```python
from build123d import *

# Parameters (mm, degrees)
F0_W      = 800
F0_H      = 300
F0_H_2    = 200
F1_DEPTH  = 100
F2_R      = 25
F2_R_2    = 75
F3_DEPTH  = 100
F4_R      = 75
F5_DEPTH  = 150
F6_R      = 82.5
F6_R_2    = 9
F6_R_3    = 25
F7_DEPTH  = 25
F8_R      = 50
F8_R_2    = 25
F9_DEPTH  = 5
F10_R     = 75
F11_DEPTH = 25
F12_R     = 37.5
F13_DEPTH = 100
F14_R     = 92.5
F14_R_2   = 9
F14_R_3   = 37.5
F15_DEPTH = 25
F16_R     = 60
F16_R_2   = 37.5
F17_DEPTH = 5
F18_W     = 1200
F18_H     = 1000
F19_DEPTH = 100
F20_W     = 1400
F20_H     = 100
F21_DEPTH = 100
F23_DEPTH = 100


with BuildPart() as f1:
    # F0 (on Front) → F1 (new body)
    with BuildSketch(Plane.XZ):
        Polygon((400, -965), (550, -965), (550, 965), (-550, 965), (-550, -965), (-400, -965), (-400, -765), (400, -765), align=None)
        with Locations((0, -465)):
            Rectangle(F0_W, F0_H, mode=Mode.SUBTRACT)
        with Locations((0, -65)):
            Rectangle(F0_W, F0_H_2, mode=Mode.SUBTRACT)
    extrude(amount=F1_DEPTH)

    # F2 (on face) → F3 (cut)
    with BuildSketch(Plane.XZ.offset(100)):
        with Locations((-300, 125)):
            Circle(F2_R)
        with Locations((0, 425)):
            Circle(F2_R_2)
        with Locations((-300, 725)):
            Circle(F2_R)
        with Locations((300, 125)):
            Circle(F2_R)
        with Locations((300, 725)):
            Circle(F2_R)
    extrude(amount=-F3_DEPTH, mode=Mode.SUBTRACT)

    # F4 (on face) → F5 (join)
    with BuildSketch(Plane.XZ.offset(100)):
        with Locations((-455, 425)):
            Circle(F4_R)
        with Locations((455, 425)):
            Circle(F4_R)
    extrude(amount=F5_DEPTH)

    # F6 (on face) → F7 (join)
    with BuildSketch(Plane.XZ.offset(100)):
        with Locations((-300, 725)):
            Circle(F6_R)
        with Locations((-300, 662.5)):
            Circle(F6_R_2, mode=Mode.SUBTRACT)
        with Locations((-362.5, 725)):
            Circle(F6_R_2, mode=Mode.SUBTRACT)
        with Locations((-300, 725)):
            Circle(F6_R_3, mode=Mode.SUBTRACT)
        with Locations((-300, 787.5)):
            Circle(F6_R_2, mode=Mode.SUBTRACT)
        with Locations((-237.5, 725)):
            Circle(F6_R_2, mode=Mode.SUBTRACT)
        with Locations((-300, 125)):
            Circle(F6_R)
        with Locations((-300, 62.5)):
            Circle(F6_R_2, mode=Mode.SUBTRACT)
        with Locations((-362.5, 125)):
            Circle(F6_R_2, mode=Mode.SUBTRACT)
        with Locations((-300, 125)):
            Circle(F6_R_3, mode=Mode.SUBTRACT)
        with Locations((-237.5, 125)):
            Circle(F6_R_2, mode=Mode.SUBTRACT)
        with Locations((-300, 187.5)):
            Circle(F6_R_2, mode=Mode.SUBTRACT)
        with Locations((300, 725)):
            Circle(F6_R)
        with Locations((300, 662.5)):
            Circle(F6_R_2, mode=Mode.SUBTRACT)
        with Locations((237.5, 725)):
            Circle(F6_R_2, mode=Mode.SUBTRACT)
        with Locations((300, 725)):
            Circle(F6_R_3, mode=Mode.SUBTRACT)
        with Locations((362.5, 725)):
            Circle(F6_R_2, mode=Mode.SUBTRACT)
        with Locations((300, 787.5)):
            Circle(F6_R_2, mode=Mode.SUBTRACT)
        with Locations((300, 125)):
            Circle(F6_R)
        with Locations((237.5, 125)):
            Circle(F6_R_2, mode=Mode.SUBTRACT)
        with Locations((300, 62.5)):
            Circle(F6_R_2, mode=Mode.SUBTRACT)
        with Locations((300, 125)):
            Circle(F6_R_3, mode=Mode.SUBTRACT)
        with Locations((362.5, 125)):
            Circle(F6_R_2, mode=Mode.SUBTRACT)
        with Locations((300, 187.5)):
            Circle(F6_R_2, mode=Mode.SUBTRACT)
    extrude(amount=F7_DEPTH)

    # F8 (on face) → F9 (join)
    with BuildSketch(Plane.XZ.offset(125)):
        with Locations((-300, 725)):
            Circle(F8_R)
        with Locations((-300, 725)):
            Circle(F8_R_2, mode=Mode.SUBTRACT)
        with Locations((-300, 125)):
            Circle(F8_R)
        with Locations((-300, 125)):
            Circle(F8_R_2, mode=Mode.SUBTRACT)
        with Locations((300, 725)):
            Circle(F8_R)
        with Locations((300, 725)):
            Circle(F8_R_2, mode=Mode.SUBTRACT)
        with Locations((300, 125)):
            Circle(F8_R)
        with Locations((300, 125)):
            Circle(F8_R_2, mode=Mode.SUBTRACT)
    extrude(amount=F9_DEPTH)

    # F10 (on face) → F11 (join)
    with BuildSketch(Plane.XZ.offset(100)):
        with Locations((0, 425)):
            Circle(F10_R)
    extrude(amount=-F11_DEPTH)

    # F12 (on face) → F13 (cut)
    with BuildSketch(Plane.XZ.offset(100)):
        with Locations((0, 850)):
            Circle(F12_R)
    extrude(amount=-F13_DEPTH, mode=Mode.SUBTRACT)

    # F14 (on face) → F15 (join)
    with BuildSketch(Plane.XZ.offset(100)):
        with Locations((0, 850)):
            Circle(F14_R)
        with Locations((-72.5, 850)):
            Circle(F14_R_2, mode=Mode.SUBTRACT)
        with Locations((0, 777.5)):
            Circle(F14_R_2, mode=Mode.SUBTRACT)
        with Locations((0, 850)):
            Circle(F14_R_3, mode=Mode.SUBTRACT)
        with Locations((0, 922.5)):
            Circle(F14_R_2, mode=Mode.SUBTRACT)
        with Locations((72.5, 850)):
            Circle(F14_R_2, mode=Mode.SUBTRACT)
    extrude(amount=F15_DEPTH)

    # F16 (on face) → F17 (join)
    with BuildSketch(Plane.XZ.offset(125)):
        with Locations((0, 850)):
            Circle(F16_R)
        with Locations((0, 850)):
            Circle(F16_R_2, mode=Mode.SUBTRACT)
    extrude(amount=F17_DEPTH)

    # F18 (on face) → F19 (cut)
    with BuildSketch(Plane.XZ.offset(100)):
        with Locations((31.1626179577, -465)):
            Rectangle(F18_W, F18_H)
    extrude(amount=-F19_DEPTH, mode=Mode.SUBTRACT)

    # F20 (on face) → F21 (join)
    with BuildSketch(Plane(origin=(0, 0, 35), x_dir=(1, 0, 0), z_dir=(0, 0, -1))):
        with Locations((0, 50)):
            Rectangle(F20_W, F20_H)
    extrude(amount=F21_DEPTH)

    # F22 (on face) → F23 (join)
    with BuildSketch(Plane.XZ.offset(100)):
        Polygon((-600, -65), (-700, -65), (-700, -965), (-600, -965), (-600, -465), (600, -465), (600, -965), (700, -965), (700, -65), (600, -65), (600, -365), (-600, -365), align=None)
    extrude(amount=-F23_DEPTH)


solid = f1.part
```
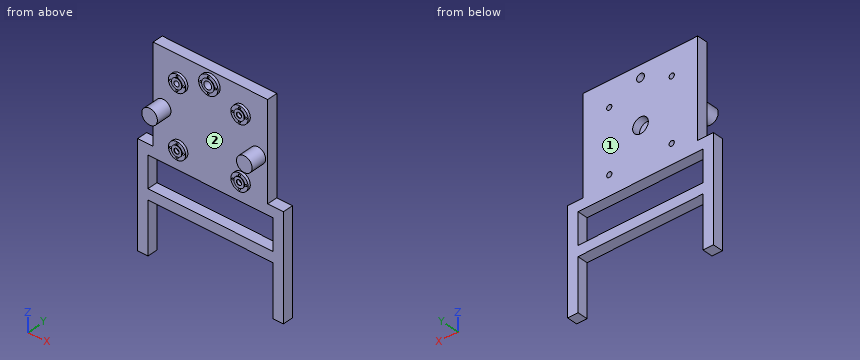
Work out the finished part from the listing and answer in its coordinate system (mm). Face numbers are marked on the shaded views. Give positions to 0.01 mm unless a question says otherwise; leave off trailing zeros. Write each loop counter-clockwise with the first axis right and the second up, starting at its lowest first coordinate (ties: lowest second). Pieces come first, ordered by that corner, then holes. Notation, with made-up numbers: (32.5, 18) -> (82.5, 18) arc R28 ccw to (82.5, 36) -> close; hole circle Ø8 at (15, 66). An arc over 180 degrees is marked (long way). Write item = value, one per line.
Q1. Section B-B on x = -455 is taken. Determine the outline of the cut face in (y, z).
Computed values:
outline = (-250, 350) -> (-100, 350) -> (-100, -65) -> (0, -65) -> (0, 965) -> (-100, 965) -> (-100, 500) -> (-250, 500) -> close; (-100, -465) -> (0, -465) -> (0, -365) -> (-100, -365) -> close
Q2. Section C-C on y = -35 is taken. Determine the outline of the cut face in (x, z).
Computed values:
outline = (-700, -965) -> (-600, -965) -> (-600, -465) -> (600, -465) -> (600, -965) -> (700, -965) -> (700, 35) -> (550, 35) -> (550, 965) -> (-550, 965) -> (-550, 35) -> (-700, 35) -> close; hole (-600, -365) -> (600, -365) -> (600, -65) -> (-600, -65) -> close; hole circle Ø50 at (-300, 125); hole circle Ø50 at (-300, 725); hole circle Ø150 at (0, 425); hole circle Ø75 at (0, 850); hole circle Ø50 at (300, 125); hole circle Ø50 at (300, 725)
Q3. For a pull along X with two mould halves and no side action, classify the marked faces 1 and 2 as pulls with the +X half, pulls with the -X half, needs draft (parallel to the pull), parting line crosses it, or undercut.
Computed values:
face_1 = needs draft
face_2 = undercut
Q4. Section D-D on y = -159.5 is taken. Determine the outline of the cut face in (x, z).
Computed values:
outline = circle Ø150 at (-455, 425); circle Ø150 at (455, 425)
Q5. Flat-ended cylindrical pins translate along their axes: pin 1 Ø16 at (x, z) = (-237.5, 725) entering from -Y; pin 2 Ø2 at (x, y) = (129.5, -35) entering from -Z; pin 3 Ø20.5 at (x, z) = (-362.5, 725) entering from -Y. Find the tip coordinate at first contact, or state that the pin passes through.
Computed values:
pin_1 = -100
pin_2 = -465
pin_3 = -125
Q6. Section A-A on z = -109 is taken. Determine the outline of the cut face in (x, y).
Computed values:
outline = (-700, -100) -> (-600, -100) -> (-600, 0) -> (-700, 0) -> close; (600, -100) -> (700, -100) -> (700, 0) -> (600, 0) -> close
Q7. Consider line 1 along Z through (x, y) = (300, -128); line 2 along Z through (x, y) = (300, -53); line 3 along Z through (x, y) = (123, -99.5). Determine where each line is inside the solid, lowest interval first.
Computed values:
line_1 = 75 to 100, 150 to 175, 675 to 700, 750 to 775
line_2 = -465 to -365, -65 to 100, 150 to 700, 750 to 965
line_3 = -465 to -365, -65 to 965
